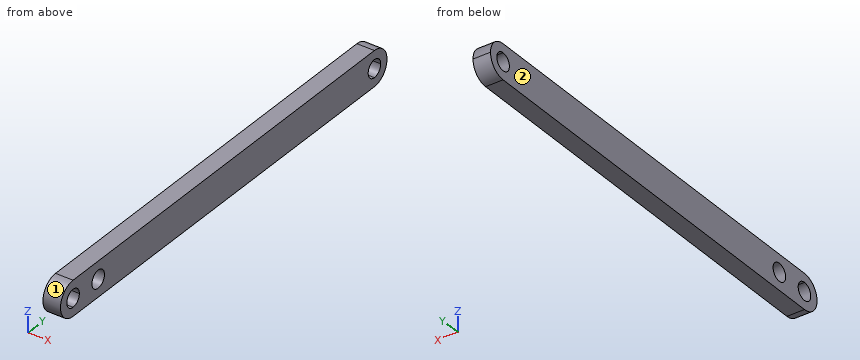
```python
from build123d import *

# Parameters (mm, degrees)
F1_DEPTH = 25.4


with BuildPart() as f1:
    # F0 (on Right) → F1 (new body)
    with BuildSketch(Plane.YZ):
        with BuildLine():
            ThreePointArc((-239.6828063071, -21.0989156985), (-247.1222940649, -3.1384034563), (-265.0828063071, 4.3010843015))
            Line((-265.0828063071, 4.3010843015), (-265.0828063071, -8.3989156985))
            ThreePointArc((-265.0828063071, -8.3989156985), (-256.102550186, -12.1186595774), (-252.3828063071, -21.0989156985))
            ThreePointArc((-252.3828063071, -21.0989156985), (-256.102550186, -30.0791718195), (-265.0828063071, -33.7989156985))
            Line((-265.0828063071, -33.7989156985), (-265.0828063071, -46.4989156985))
            ThreePointArc((-265.0828063071, -46.4989156985), (-247.1222940649, -39.0594279406), (-239.6828063071, -21.0989156985))
        make_face()
        with BuildLine():
            Line((344.5171936929, 4.3010843015), (-265.0828063071, 4.3010843015))
            ThreePointArc((-265.0828063071, 4.3010843015), (-247.1222940649, -3.1384034563), (-239.6828063071, -21.0989156985))
            ThreePointArc((-239.6828063071, -21.0989156985), (-247.1222940649, -39.0594279406), (-265.0828063071, -46.4989156985))
            Line((-265.0828063071, -46.4989156985), (344.5171936929, -46.4989156985))
            ThreePointArc((344.5171936929, -46.4989156985), (319.1171936929, -21.0989156985), (344.5171936929, 4.3010843015))
        make_face()
        with BuildLine():
            ThreePointArc((-201.5828063071, -21.0989156985), (-214.2828063071, -33.7989156985), (-226.9828063071, -21.0989156985))
            ThreePointArc((-226.9828063071, -21.0989156985), (-214.2828063071, -8.3989156985), (-201.5828063071, -21.0989156985))
        make_face(mode=Mode.SUBTRACT)
        with BuildLine():
            Line((-265.0828063071, -8.3989156985), (-265.0828063071, 4.3010843015))
            ThreePointArc((-265.0828063071, 4.3010843015), (-290.4828063071, -21.0989156985), (-265.0828063071, -46.4989156985))
            Line((-265.0828063071, -46.4989156985), (-265.0828063071, -33.7989156985))
            ThreePointArc((-265.0828063071, -33.7989156985), (-277.7828063071, -21.0989156985), (-265.0828063071, -8.3989156985))
        make_face()
        with BuildLine():
            ThreePointArc((369.9171936929, -21.0989156985), (362.4777059351, -3.1384034563), (344.5171936929, 4.3010843015))
            Line((344.5171936929, 4.3010843015), (344.5171936929, -8.3989156985))
            ThreePointArc((344.5171936929, -8.3989156985), (353.497449814, -12.1186595774), (357.2171936929, -21.0989156985))
            ThreePointArc((357.2171936929, -21.0989156985), (353.497449814, -30.0791718195), (344.5171936929, -33.7989156985))
            Line((344.5171936929, -33.7989156985), (344.5171936929, -46.4989156985))
            ThreePointArc((344.5171936929, -46.4989156985), (362.4777059351, -39.0594279406), (369.9171936929, -21.0989156985))
        make_face()
        with BuildLine():
            Line((344.5171936929, -8.3989156985), (344.5171936929, 4.3010843015))
            ThreePointArc((344.5171936929, 4.3010843015), (319.1171936929, -21.0989156985), (344.5171936929, -46.4989156985))
            Line((344.5171936929, -46.4989156985), (344.5171936929, -33.7989156985))
            ThreePointArc((344.5171936929, -33.7989156985), (331.8171936929, -21.0989156985), (344.5171936929, -8.3989156985))
        make_face()
    extrude(amount=F1_DEPTH)


solid = f1.part
```
The listing builds one solid part. Answer for the finished solid, in the listing's coordinates (mm). Face numbers are marked on the shaded views. Round coordinates to 2 decimals unless told otherwise and drop trailing zeros. Write each loop counter-clockwise with the first axis right and the second up, starting at its lowest first coordinate (ties: lowest second). Pieces come first, ordered by that corner, then holes. Notation, with made-up numbers: (61.5, 56.5) -> (88.5, 56.5) arc R24 cw to (88.5, 91.5) -> close; hole circle Ø7 at (43, 71). An arc over 180 degrees is marked (long way). Answer as a JSON object with one key per item and string values. Group by question number.
Q1. Straight lines are drawn through the part: line 1 along Y through (x, z) = (6, -19); line 2 along Y through (x, z) = (10.75, -9.5); line 3 along Z through (x, y) = (4.25, -261). For each, find the intervals that lie inside material, in ascending order.
Q2. Section A-A (x = 15.5) is taken. Write down the section's boundary in (y, z).
Q3. Each of these flat-tipped pins is pushed along its axis until it touches: pin 1 Ø1.5 at (x, z) = (20.5, -39.5) entering from +Y; pin 2 Ø23 at (y, z) = (-214.28, -21.1) entering from -X; pin 3 Ø5 at (x, z) = (7.5, -40) entering from +Y; pin 4 Ø1 at (x, z) = (21, -8.5) entering from -Y. Where does it stop, or does it pass through?
Q4. Determine the mould class of the marked faces 1 and 2 for opening direction Z: pulls with the +Z half, pulls with the -Z half, needs draft (parallel to the pull), parting line crosses it, or undercut.
Check values:
{
 "1": {"line 1": "-290.4 to -277.61, -252.56 to -226.81, -201.76 to 331.99, 357.04 to 369.83", "line 2": "-287.68 to -270.26, -259.91 to -219.46, -209.11 to 339.34, 349.69 to 367.11", "line 3": "-46.5 to -33.12, -9.07 to 4.3"},
 "2": {"outline": "(-265.08, -46.5) -> (344.52, -46.5) arc R25.4 ccw to (344.52, 4.3) -> (-265.08, 4.3) arc R25.4 ccw to start; hole circle Ø25.4 at (-265.08, -21.1); hole circle Ø25.4 at (-214.28, -21.1); hole circle Ø25.4 at (344.52, -21.1)"},
 "3": {"pin 1": "y = 362.78", "pin 2": "through", "pin 3": "y = 363.91", "pin 4": "y = -287.42"},
 "4": {"face 1": "parting line crosses it", "face 2": "needs draft"}
}
